Read the model definition and answer for the solid it produces. Units are mm, in the model's axes. Coordinates: 2 decimals unless noted, no trailing zeros. Loops run counter-clockwise (first coordinate to the right, second up) from the corner with the lowest first, then second, coordinate; pieces in that order, holes last. Notation, with made-up numbers: (-18.5, 27) - (9.5, 27) arc R19 cw to (9.5, 33) - close; hole circle Ø5 at (19, -30.5). An arc over 180 degrees is marked (long way). Use one line per item in the form item = value. Start each with the question number.
1) A cutting plane is placed at A-A (x = -50). Give the vertices of the cut face in (y, z).
2) Each of these flat-tipped pins is pushed along its axis until it touches: P1, Ø7, axis at x = 50, z = 0, coming from the -Y side; P2, Ø4.5, axis at x = -50, z = -75, coming from the -Y side. Where does it stop, or does it pass through?
3) Consider line 1 (X direction, y = -0.4, z = 104.5); line 2 (Z direction, x = -50, y = 0.9). Determine where each line is inside the solid, lowest interval first.
4) The mould has two halves that part along X. Classify faces 1 (the face through (2, 1.588, 2)), 2 (the face through (-52.732, -0.022, -75.359)): released by +X, released by -X, zero draft, split by the parting line, or undercut.
5) A cutting plane is placed at B-B (z = 75). Give the vertices of the cut face in (x, y), and give its area (3 significant figures).
Autodesk Inventor part; units mm, degrees
ref_plane "YZ Plane" through (0, 0, 0) normal (1, 0, 0) x (0, 1, 0)
ref_plane "XZ Plane" through (0, 0, 0) normal (0, 1, 0) x (-1, 0, 0)
ref_plane "XY Plane" through (0, 0, 0) normal (0, 0, 1) x (1, 0, 0)
sketch "Sketch1" plane through (0, 0, 0) normal (0, 1, 0) x (-1, 0, 0)
  line L0 (109.5, 109.5) -> (-109.5, 109.5)
  line L1 (-109.5, 109.5) -> (-109.5, -109.5)
  line L2 (-109.5, -109.5) -> (109.5, -109.5)
  line L3 (109.5, -109.5) -> (109.5, 109.5)
  line L4 (109.5, 109.5) -> (-109.5, -109.5) construction
  line L5 (-109.5, 109.5) -> (109.5, -109.5) construction
  point P0 (0, 0)
  dimension "d0" = 219
extrude "Extrusion1" add sketch "Sketch1" along normal mid plane 3.175
chamfer "Chamfer1" distance 4 angle 45 4 edges at (-109.5, 0, 109.5) (-109.5, 0, -109.5) (109.5, 0, -109.5) (109.5, 0, 109.5)
sketch "Sketch3" plane through (0, 1.5875, 0) normal (0, 1, 0) x (1, 0, 0)
  line L0 (-104.5, -104.5) -> (104.5, -104.5) construction
  line L1 (104.5, -104.5) -> (104.5, 104.5) construction
  line L2 (104.5, 104.5) -> (-104.5, 104.5) construction
  line L3 (-104.5, 104.5) -> (-104.5, -104.5) construction
  line L4 (-104.5, -104.5) -> (104.5, 104.5) construction
  line L5 (104.5, -104.5) -> (-104.5, 104.5) construction
  line L6 (-78.5, 50) -> (-46.5, 50) construction
  line L7 (-78.5, -50) -> (-46.5, -50) construction
  line L8 (46.5, 0) -> (78.5, 0) construction
  point P0 (0, 0)
  point P1 (0, 0)
  dimension "d16" = 209
  dimension "d17" = 209
  dimension "d18" = 32
  dimension "d20" = 46.5
  dimension "d21" = 46.5
  dimension "d22" = 100
  dimension "d23" = 50
  dimension "d24" = 93
hole "Hole1" at (-104.5, 1.5875, -104.5) at (104.5, 1.5875, -104.5) at (104.5, 1.5875, 104.5) at (-104.5, 1.5875, 104.5) direction (0, -1, 0) diameter 3.2 end through all
sketch "Sketch4" plane through (0, 1.5875, 0) normal (0, 1, 0) x (1, 0, 0)
  line L0 (1.5, 22.5) -> (1.5, -22.5)
  line L1 (-109.5, 105.5) -> (-109.5, -105.5)
  point P0 (0, 0)
  point P1 (1.5, 0)
  point P2 (-50, 75)
  point P3 (50, 0)
  point P4 (-50, -75)
  dimension "d38" = 45
  dimension "d39" = 111
  dimension "d52" = 150
  dimension "d53" = 75
  dimension "d54" = 100
  dimension "d55" = 50
hole "Hole2" at (-50, 1.5875, 75) at (-50, 1.5875, -75) at (50, 1.5875, 0) direction (0, -1, 0) diameter 5.5118 depth 6.4
properties part number "Y-Carriage_Plate_LM3033_v2" material "Aluminum 6061"
Found:
q1.outline = (-1.59, -109.5) - (1.59, -109.5) - (1.59, -77.76) - (-1.59, -77.76) - close; (-1.59, -72.24) - (1.59, -72.24) - (1.59, 72.24) - (-1.59, 72.24) - close; (-1.59, 77.76) - (1.59, 77.76) - (1.59, 109.5) - (-1.59, 109.5) - close
q2.P1 = -1.59
q2.P2 = through
q3.line_1 = -109.5 to -106.1, -102.9 to 102.9, 106.1 to 109.5
q3.line_2 = -109.5 to -77.76, -72.24 to 72.24, 77.76 to 109.5
q4.face_1 = zero draft
q4.face_2 = undercut
q5.outline = (-109.5, -1.59) - (-52.76, -1.59) - (-52.76, 1.59) - (-109.5, 1.59) - close; (-47.24, -1.59) - (109.5, -1.59) - (109.5, 1.59) - (-47.24, 1.59) - close
q5.area = 678 mm^2
